```python
from build123d import *

# Parameters (mm, degrees)
SKETCH1_W           = 130
SKETCH1_H           = 130
BOSS_EXTRUDE1_DEPTH = 5
SKETCH2_R           = 1.5
CUT_EXTRUDE1_DEPTH  = 5
SKETCH3_R           = 1.5
CUT_EXTRUDE2_DEPTH  = 5
SKETCH4_R           = 1.5
CUT_EXTRUDE3_DEPTH  = 5
SKETCH5_W           = 20
SKETCH5_H           = 20
CUT_EXTRUDE4_DEPTH  = 5


with BuildPart() as part:
    # Sketch1 → Boss-Extrude1 (new body)
    with BuildSketch(Plane(origin=(0, 0, 0), x_dir=(1, 0, 0), z_dir=(0, 1, 0))):
        Rectangle(SKETCH1_W, SKETCH1_H)
    extrude(amount=BOSS_EXTRUDE1_DEPTH)

    # Sketch2 → Cut-Extrude1 (cut)
    with BuildSketch(Plane.XZ):
        with Locations(Location((19.9, 55.5, 0), (0, 0, 270))):
            Circle(SKETCH2_R)
        with Locations(Location((19.9, 18.5, 0), (0, 0, 270))):
            Circle(SKETCH2_R)
    extrude(amount=-CUT_EXTRUDE1_DEPTH, mode=Mode.SUBTRACT)

    # Sketch3 → Cut-Extrude2 (cut)
    with BuildSketch(Plane(origin=(0, 5, 0), x_dir=(1, 0, 0), z_dir=(0, 1, 0))):
        with Locations(Location((-28.25, 15.5, 0), (0, 0, 270))):
            Circle(SKETCH3_R)
        with Locations(Location((28.25, 15.5, 0), (0, 0, 270))):
            Circle(SKETCH3_R)
    extrude(amount=-CUT_EXTRUDE2_DEPTH, mode=Mode.SUBTRACT)

    # Sketch4 → Cut-Extrude3 (cut)
    with BuildSketch(Plane(origin=(0, 5, 0), x_dir=(1, 0, 0), z_dir=(0, 1, 0))):
        with Locations(Location((-60, 50, 0), (0, 0, 270))):
            Circle(SKETCH4_R)
        with Locations(Location((60, 50, 0), (0, 0, 270))):
            Circle(SKETCH4_R)
        with Locations(Location((60, -50, 0), (0, 0, 270))):
            Circle(SKETCH4_R)
        with Locations(Location((-60, -50, 0), (0, 0, 270))):
            Circle(SKETCH4_R)
    extrude(amount=-CUT_EXTRUDE3_DEPTH, mode=Mode.SUBTRACT)

    # Sketch5 → Cut-Extrude4 (cut)
    with BuildSketch(Plane(origin=(0, 5, 0), x_dir=(1, 0, 0), z_dir=(0, 1, 0))):
        with Locations((-35, -18)):
            Rectangle(SKETCH5_W, SKETCH5_H)
    extrude(amount=-CUT_EXTRUDE4_DEPTH, mode=Mode.SUBTRACT)


solid = part.part
```
Part model, mm, in its own coordinate system. A direction names the side the tool comes from. Coordinates: 2 decimals unless noted, no trailing zeros. Write each loop counter-clockwise with the first axis right and the second up, starting at its lowest first coordinate (ties: lowest second). Pieces come first, ordered by that corner, then holes.
Item 1: Slice it at A-A (x = 28.25). Write the cut outline in (y, z).
Item 2: Which spindle directions (+Z, -Z, +X, -X, +Y, -Y) get a long thin tool onto all of the face, cutting with end or side? Do faces 4 (the face through (-1, 2, 65)), 5 (the face through (-35, 3, 8)). Say none if no direction does.
Item 3: Slice it at C-C (x = -60). Write the cut outline in (y, z).
Item 4: Slice it at B-B (z = 18.5). Write the cut outline in (x, y), and give its area (3 significant figures).
Item 5: Slice it at D-D (y = 2.9). Count the separate pieces of the cut face and the enclosed holes in it, and give its area (3 significant figures).
Item 6: Mould opens along X. For faces 1 (the face through (-45, 3, 18)), 2 (the face through (-65, 2, 1)), 3 (the face through (-1, 2, -65)) say: released by +X, released by -X, zero draft, split by the parting line, or undercut.
Item 7: Probe line 1 (X direction, y = 2.4, z = 50); line 2 (X direction, y = 4.2, z = 22); line 3 (X direction, y = 2.55, z = -15.5). List the from-to ranges inside material, lowest first.
Results found:
1. outline: (0, -65) - (5, -65) - (5, -17) - (0, -17) - close; (0, -14) - (5, -14) - (5, 65) - (0, 65) - close
2. face 4: +Z, +X, -X, +Y, -Y
2. face 5: +Y, -Y
3. outline: (0, -65) - (5, -65) - (5, -51.5) - (0, -51.5) - close; (0, -48.5) - (5, -48.5) - (5, 48.5) - (0, 48.5) - close; (0, 51.5) - (5, 51.5) - (5, 65) - (0, 65) - close
4. outline: (-65, 0) - (-45, 0) - (-45, 5) - (-65, 5) - close; (-25, 0) - (18.4, 0) - (18.4, 5) - (-25, 5) - close; (21.4, 0) - (65, 0) - (65, 5) - (21.4, 5) - close
4. area: 535 mm2
5. separate pieces: 1
5. enclosed holes: 9
5. area: 16,400 mm2
6. face 1: undercut
6. face 2: released by -X
6. face 3: zero draft
7. line 1: x = -65 to -61.5, -58.5 to 58.5, 61.5 to 65
7. line 2: x = -65 to -45, -25 to 65
7. line 3: x = -65 to -29.75, -26.75 to 26.75, 29.75 to 65
